Here's how the part is built. I have some questions about the finished solid (model axes, mm). A direction names the side the tool comes from. Give positions to 0.01 mm unless a question says otherwise; leave off trailing zeros. Write each loop counter-clockwise with the first axis right and the second up, starting at its lowest first coordinate (ties: lowest second). Pieces come first, ordered by that corner, then holes. Notation, with made-up numbers: M 77.5,-1.5 L 105.5,-1.5 A18 ccw 105.5,11.5 Z; hole C 49,-24 d10. An arc over 180 degrees is marked long. Answer as CSV lines item,"result". Start each with the question number.
Q1. If I drill on line 1 along Y through (x, z) = (-5, 2.5); line 2 along Y through (x, z) = (-0.5, 1.5); line 3 along X through (y, z) = (15, 3.25), over which ranges is the centre line in solid material (lowest first)?
Q2. On a 3-axis mill with a long thin cutter (end or side, diameter ignored), from which of +Z, -Z, +X, -X, +Y, -Y can I reach the whole of each face in a straight line? I mean faces 1 (the flat face through (0, 22.188, 3)), 2 (the flat face through (0, 13.044, 5)). Say none if no direction works.
Q3. Suppose I cut it at D-D (x = -2). Write out the boundary of the cut face in (y, z), then the cut area to 3 significant figures.
Q4. Suppose I cut it at B-B (z = 2.5). Write out the boundary of the cut face in (x, y), then the cut area to 3 significant figures.
Q5. Suppose I cut it at C-C (y = 19). Write out the boundary of the cut face in (x, z), then the cut area to 3 significant figures.
Q6. For pin 1 (2 mm diameter, centred on y = 10, z = 3, fed in from -X); pin 2 (1.5 mm diameter, centred on x = -2.5, z = 2, fed in from +Y); pin 3 (5 mm diameter, centred on x = -0.5, y = 14.5, fed in from -Z), each with a flat end and sliding along its axis, tell me the tip position at first contact or that it passes through.
Q7. Suppose I cut it at A-A (x = 3.25). Write out the boundary of the cut face in (y, z).
Autodesk Inventor part; units mm, degrees
ref_plane "YZ Plane" through (0, 0, 0) normal (1, 0, 0) x (0, 1, 0)
ref_plane "XZ Plane" through (0, 0, 0) normal (0, 1, 0) x (-1, 0, 0)
ref_plane "XY Plane" through (0, 0, 0) normal (0, 0, 1) x (1, 0, 0)
sketch "Sketch1" plane through (0, 0, 0) normal (0, 0, 1) x (1, 0, 0)
  line L0 (-5.9795, 4.5091) -> (6.9237, 4.5091)
  line L1 (6.9237, 4.5091) -> (6.9237, -8.8513)
  line L2 (6.9237, -8.8513) -> (-5.9795, -8.8513)
  line L3 (-5.9795, -8.8513) -> (-5.9795, 4.5091)
  point P0 (0, 0)
  dimension "d0" = 12.9032
  dimension "d1" = 13.3604
extrude "Extrusion1" add sketch "Sketch1" along normal blind 6.9342
sketch "Sketch2" plane through (-5.9795, 4.5091, 0) normal (0, 1, 0) x (1, 0, 0)
  circle A0 centre (6.4761, -3.3308) radius 3.2234
  point P0 (5.9795, 0)
  dimension "d4" = 6.4469
extrude "Extrusion2" add sketch "Sketch2" along normal blind 8.5344
sketch "Sketch3" plane through (0.4966, 13.0435, 3.3308) normal (0, 1, 0) x (1, 0, 0)
  circle A0 centre (0, 0) radius 1.27
  point P0 (-0.4966, 3.3308)
  dimension "d7" = 2.54
extrude "Extrusion3" add sketch "Sketch3" along normal blind 9.144
sketch "Sketch4" plane through (-5.9795, -8.8513, 0) normal (-1, 0, 0) x (0, 0, 1)
  point P0 (0, 8.8513)
properties part number "Aidan Sherry Switch"
Resolved:
1,line 1,"-8.85 to 4.51"
1,line 2,"-8.85 to 13.04"
1,line 3,"-0.77 to 1.76"
2,face 1,"+Z, -Z, +X, -X, +Y"
2,face 2,"+Y"
3,outline,"M -8.85,0 L 4.51,0 L 4.51,1.29 L 13.04,1.29 L 13.04,5.37 L 4.51,5.37 L 4.51,6.93 L -8.85,6.93 Z"
3,area,"127 mm^2"
4,outline,"M -5.98,-8.85 L 6.92,-8.85 L 6.92,4.51 L 3.61,4.51 L 3.61,13.04 L 1.46,13.04 L 1.46,22.19 L -0.46,22.19 L -0.46,13.04 L -2.62,13.04 L -2.62,4.51 L -5.98,4.51 Z"
4,area,"243 mm^2"
5,outline,"C 0.5,3.33 d2.54"
5,area,"5.07 mm^2"
6,pin 1,"x = -2.73"
6,pin 2,"y = 13.04"
6,pin 3,"z = 0.11"
7,outline,"M -8.85,0 L 4.51,0 L 4.51,1.65 L 13.04,1.65 L 13.04,5.01 L 4.51,5.01 L 4.51,6.93 L -8.85,6.93 Z"
